Read the model definition and answer for the solid it produces. Units are mm, in the model's axes. Face numbers are marked on the shaded views. A direction names the side the tool comes from. Give positions to 0.01 mm unless a question says otherwise; leave off trailing zeros. Write each loop counter-clockwise with the first axis right and the second up, starting at its lowest first coordinate (ties: lowest second). Pieces come first, ordered by that corner, then holes. Notation, with made-up numbers: M 55,-2.5 L 76,-2.5 A26 ccw 76,23.5 Z; hole C -9,7 d6. An arc over 180 degrees is marked long. Put each result on its own line as item: value.
from build123d import *

# Parameters (mm, degrees)
SKETCH1_R           = 10
SKETCH1_R_2         = 3
BOSS_EXTRUDE1_DEPTH = 15
CUT_EXTRUDE1_START  = -2
SKETCH2_R           = 10.003270656
SKETCH2_R_2         = 7.618419173
CUT_EXTRUDE1_DEPTH  = 11


with BuildPart() as part:
    # Sketch1 → Boss-Extrude1 (new body)
    with BuildSketch(Plane.XY):
        Circle(SKETCH1_R)
        Circle(SKETCH1_R_2, mode=Mode.SUBTRACT)
    extrude(amount=BOSS_EXTRUDE1_DEPTH)

    # Sketch2 → Cut-Extrude1 (cut)
    with BuildSketch(Plane.XY.offset(15).offset(CUT_EXTRUDE1_START)):
        Circle(SKETCH2_R)
        Circle(SKETCH2_R_2, mode=Mode.SUBTRACT)
    extrude(amount=-CUT_EXTRUDE1_DEPTH, mode=Mode.SUBTRACT)


solid = part.part
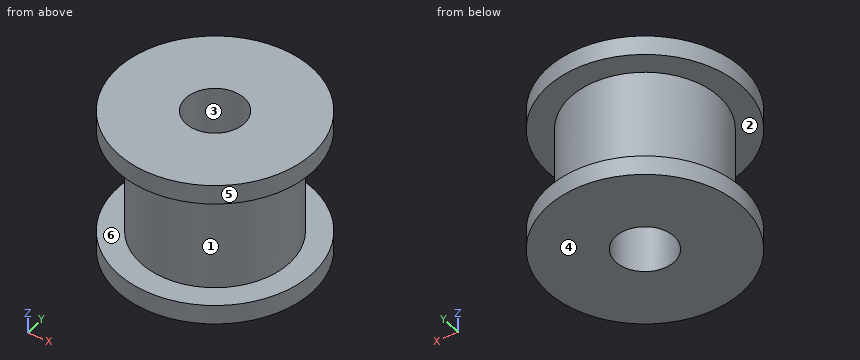
(1) Section B-B on x = 0 is taken. Determine the outline of the cut face in (y, z), and give its area (3 significant figures).
Result:
outline: M -10,0 L -3,0 L -3,15 L -10,15 L -10,13 L -7.62,13 L -7.62,2 L -10,2 Z; M 3,0 L 10,0 L 10,2 L 7.62,2 L 7.62,13 L 10,13 L 10,15 L 3,15 Z
area: 158 mm²
(2) Given pin 1 Ø4 at (x, y) = (4, 0.5) entering from -Z, flat-ended and moving along its own axis, determine where the tip first touches the part or whether it passes through.
Result:
pin 1: stops at z = 0
(3) Section D-D on z = 8.25 is taken. Determine the outline of the cut face in (x, y), and give its area (3 significant figures).
Result:
outline: C 0,0 d15.24; hole C 0,0 d6
area: 154 mm²
(4) Straight lines are drawn through the part: line 1 along Z through (x, y) = (6.25, -6.25); line 2 along Y through (x, z) = (0, 5); line 3 along X through (y, z) = (2, 3). For each, find the intervals that lie inside material, in ascending order. Write a range as from..to.
Result:
line 1: z = 0..2, 13..15
line 2: y = -7.62..-3, 3..7.62
line 3: x = -7.35..-2.24, 2.24..7.35
(5) For a pull along Z with two mould halves and no side action, classify the marked faces 1, 2, 3 and 4 as +Z half, -Z half, draft (parallel to the pull), parting line (faces both ways), or undercut.
Result:
face 1: undercut
face 2: undercut
face 3: draft
face 4: -Z half
(6) Section A-A on y = 8 is taken. Determine the outline of the cut face in (x, z), and give its area (3 significant figures).
Result:
outline: M -6,0 L 6,0 L 6,2 L -6,2 Z; M -6,13 L 6,13 L 6,15 L -6,15 Z
area: 48.0 mm²
(7) Which of the six approach directions +Z, -Z, +X, -X, +Y, -Y give full straight-line access (tool end or side, diameter ignored) to the marked faces 5 and 6?
Result:
face 5: +Z, -Z
face 6: none
